Geometry: see drawing. Coordinates: mm, zero at the bounding-box minimum. A direction names the side the tool comes from. Round coordinates to 2 decimals unless told otherwise and drop trailing zeros. Loops run counter-clockwise (first coordinate to the right, second up) from the corner with the lowest first, then second, coordinate; pieces in that order, holes last. Notation, with made-up numbers: (75, -38.5) - (97, -38.5) arc R6 cw to (97, -34.5) - close; hole circle Ø7 at (24, 22). An arc over 180 degrees is marked (long way). Write item = value, one per line. Start each with the question number.
Item 1: Line query: line 1 (Y direction, x = 28.7, z = 30) (1 decimal); line 2 (Y direction, x = 33, z = 30) (3 decimals); line 3 (Z direction, x = 32, y = 30). Output: solid intervals per line, ascending. Write a range as from..to.
Item 2: Section C-C (z = 51). Return loops of the section in (x, y).
Item 3: Section B-B (y = 38.56). Return loops of the section in (x, z).
Item 4: Access query for the marked faces 1, 2 and 3. Directions: +Z, -Z, +X, -X, +Y, -Y. A direction counts if a zero-diameter tool reaches every point of the face in a straight line with its end or side. Return the directions, or none.
Item 5: Section D-D (x = 25). Return loops of the section in (y, z), plus the area to 3 significant figures.
Item 6: First-contact query: pin 1 (6.5 mm diameter, centred on x = 16, z = 18, fed in from -Y); pin 2 (5 mm diameter, centred on x = 35, y = 10, fed in from -Z) (3 decimals); pin 3 (1 mm diameter, centred on y = 89.5, z = 18.5, fed in from -X); pin 4 (12 mm diameter, centred on y = 21.56, z = 30, fed in from +X). Flat tips, straight axial feed; report the tip coordinate or a pass-through.
Item 7: Section A-A (x = 35). Return loops of the section in (y, z) (3 decimals).
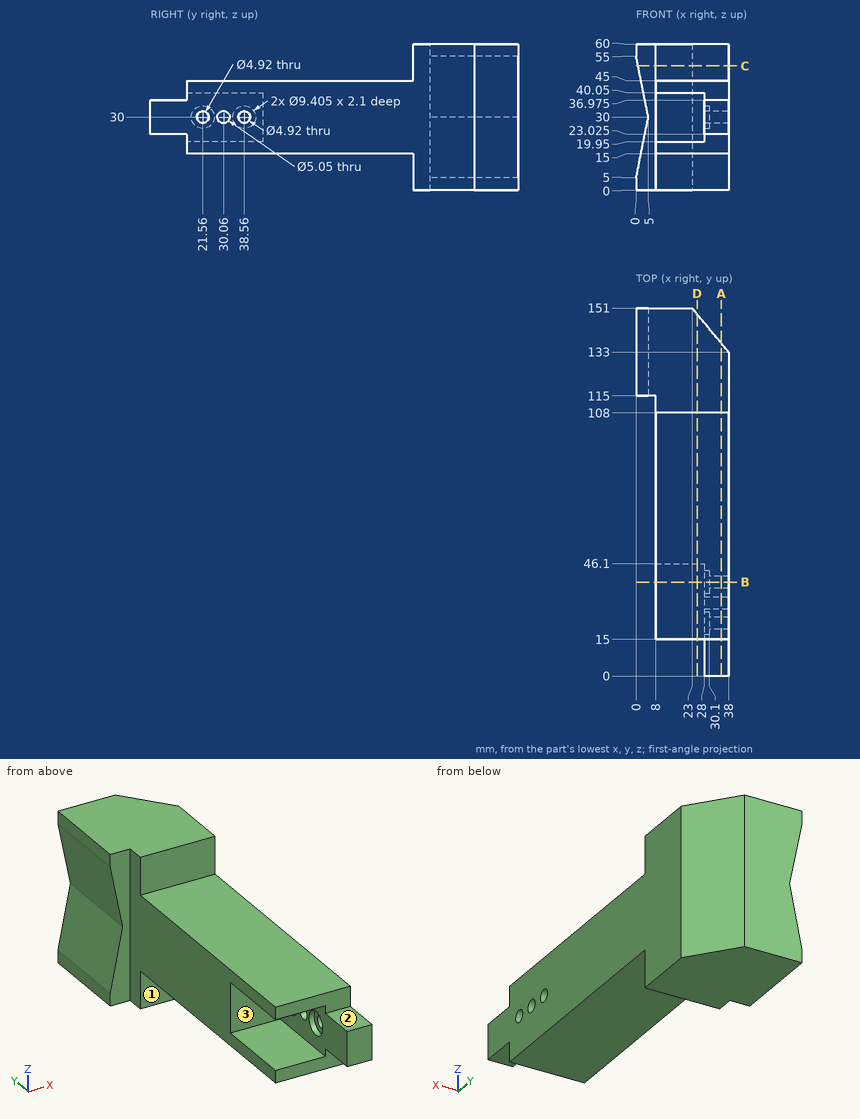
Taken from the geometry:
q1.line_1 = 0..16.9, 26.3..27.5, 32.6..33.9, 43.3..144.2
q1.line_2 = 0..19.1, 24.02..27.535, 32.585..36.1, 41.02..139
q1.line_3 = 15..27.48, 32.52..45
q2.outline = (0.8, 115) - (8, 115) - (8, 108) - (38, 108) - (38, 133) - (23, 151) - (0.8, 151) - close
q3.outline = (8, 15) - (38, 15) - (38, 27.54) - (30.1, 27.54) - (30.1, 25.3) - (28, 25.3) - (28, 19.95) - (8, 19.95) - close; (8, 40.05) - (28, 40.05) - (28, 34.7) - (30.1, 34.7) - (30.1, 32.46) - (38, 32.46) - (38, 45) - (8, 45) - close
q4.face_1 = -Z, +X, -X, -Y
q4.face_2 = +Z, +X, -X, -Y
q4.face_3 = -X, -Y
q5.outline = (15, 15) - (108, 15) - (108, 0) - (148.6, 0) - (148.6, 60) - (108, 60) - (108, 45) - (15, 45) - (15, 40.05) - (46.1, 40.05) - (46.1, 19.95) - (15, 19.95) - close
q5.area = 4,600 mm^2
q6.pin_1 = 15
q6.pin_2 = 23.025
q6.pin_3 = 8
q6.pin_4 = 38
q7.outline = (0, 23.025) - (15, 23.025) - (15, 15) - (108, 15) - (108, 0) - (136.6, 0) - (136.6, 60) - (108, 60) - (108, 45) - (15, 45) - (15, 36.975) - (0, 36.975) - close; hole circle Ø4.92 at (21.56, 30); hole circle Ø5.05 at (30.06, 30); hole circle Ø4.92 at (38.56, 30)
